from build123d import *

# Parameters (mm, degrees)
SKETCH2_W           = 50
SKETCH2_H           = 50
BOSS_EXTRUDE1_DEPTH = 50
CUT_EXTRUDE2_REACH  = 88.603
SKETCH5_R           = 2.1
CUT_EXTRUDE3_REACH  = 88.603
SKETCH6_R           = 15.5


with BuildPart() as part:
    # Sketch2 → Boss-Extrude1 (new body)
    with BuildSketch(Plane.XY):
        with Locations((25, 25)):
            Rectangle(SKETCH2_W, SKETCH2_H)
    extrude(amount=BOSS_EXTRUDE1_DEPTH)

    # Sketch5 → Cut-Extrude2 (cut, up to next)
    with BuildSketch(Plane(origin=(0, 50, 0), x_dir=(1, 0, 0), z_dir=(0, 1, 0)), mode=Mode.PRIVATE) as cut_extrude2_sk1:
        with Locations(Location((7.5, -7.5, 0), (0, 0, 270))):
            Circle(SKETCH5_R)
    cut_extrude2_tool1 = extrude(cut_extrude2_sk1.sketch, amount=-CUT_EXTRUDE2_REACH, mode=Mode.PRIVATE) & part.part
    # Sketch5 → Cut-Extrude2 (cut, up to next)
    with BuildSketch(Plane(origin=(0, 50, 0), x_dir=(1, 0, 0), z_dir=(0, 1, 0)), mode=Mode.PRIVATE) as cut_extrude2_sk2:
        with Locations(Location((42.5, -7.5, 0), (0, 0, 270))):
            Circle(SKETCH5_R)
    cut_extrude2_tool2 = extrude(cut_extrude2_sk2.sketch, amount=-CUT_EXTRUDE2_REACH, mode=Mode.PRIVATE) & part.part
    # Sketch5 → Cut-Extrude2 (cut, up to next)
    with BuildSketch(Plane(origin=(0, 50, 0), x_dir=(1, 0, 0), z_dir=(0, 1, 0)), mode=Mode.PRIVATE) as cut_extrude2_sk3:
        with Locations(Location((7.5, -42.5, 0), (0, 0, 270))):
            Circle(SKETCH5_R)
    cut_extrude2_tool3 = extrude(cut_extrude2_sk3.sketch, amount=-CUT_EXTRUDE2_REACH, mode=Mode.PRIVATE) & part.part
    # Sketch5 → Cut-Extrude2 (cut, up to next)
    with BuildSketch(Plane(origin=(0, 50, 0), x_dir=(1, 0, 0), z_dir=(0, 1, 0)), mode=Mode.PRIVATE) as cut_extrude2_sk4:
        with Locations(Location((42.5, -42.5, 0), (0, 0, 270))):
            Circle(SKETCH5_R)
    cut_extrude2_tool4 = extrude(cut_extrude2_sk4.sketch, amount=-CUT_EXTRUDE2_REACH, mode=Mode.PRIVATE) & part.part
    add(cut_extrude2_tool1.solids().sort_by_distance((7.5, 50, 7.5))[0], mode=Mode.SUBTRACT)
    add(cut_extrude2_tool2.solids().sort_by_distance((42.5, 50, 7.5))[0], mode=Mode.SUBTRACT)
    add(cut_extrude2_tool3.solids().sort_by_distance((7.5, 50, 42.5))[0], mode=Mode.SUBTRACT)
    add(cut_extrude2_tool4.solids().sort_by_distance((42.5, 50, 42.5))[0], mode=Mode.SUBTRACT)

    # Sketch6 → Cut-Extrude3 (cut, up to next)
    with BuildSketch(Plane(origin=(0, 50, 0), x_dir=(-1, 0, 0), z_dir=(0, 1, 0)), mode=Mode.PRIVATE) as cut_extrude3_sk1:
        with Locations(Location((-25, 25, 0), (0, 0, 90))):
            Circle(SKETCH6_R)
    cut_extrude3_tool1 = extrude(cut_extrude3_sk1.sketch, amount=-CUT_EXTRUDE3_REACH, mode=Mode.PRIVATE) & part.part
    add(cut_extrude3_tool1.solids().sort_by_distance((25, 50, 25))[0], mode=Mode.SUBTRACT)


solid = part.part
Input: part model. Units: mm. Frame: model coordinates. Give positions to 0.01 mm unless a question says otherwise; leave off trailing zeros. Write each loop counter-clockwise with the first axis right and the second up, starting at its lowest first coordinate (ties: lowest second). Pieces come first, ordered by that corner, then holes. Notation, with made-up numbers: M 15,2 L 37,2 A23 cw 37,10 Z; hole C 40,69 d3. An arc over 180 degrees is marked long. Use one line per item in the form item = value.
1. First-contact query: P1, Ø4, axis at x = 7.5, z = 7.5, coming from the +Y side. Flat tip, straight axial feed; report the tip coordinate or a pass-through.
Outcome:
P1 = through
2. Ray query, L1, parallel to X at y = 23, z = 7.5; L2, parallel to Z at x = 9, y = 48; L3, parallel to X at y = 31, z = 42. Return the intervals inside material, ascending.
Outcome:
L1 = 0 to 5.4, 9.6 to 40.4, 44.6 to 50
L2 = 0 to 6.03, 8.97 to 41.03, 43.97 to 50
L3 = 0 to 5.46, 9.54 to 40.46, 44.54 to 50
3. Cut plane C-C on x = 25. Return loops of the section in (y, z), and give its area (3 significant figures).
Outcome:
outline = M 0,0 L 50,0 L 50,9.5 L 0,9.5 Z; M 0,40.5 L 50,40.5 L 50,50 L 0,50 Z
area = 950 mm²
4. Cut plane A-A on z = 42.5. Return loops of the section in (x, y), and give its area (3 significant figures).
Outcome:
outline = M 0,0 L 5.4,0 L 5.4,50 L 0,50 Z; M 9.6,0 L 40.4,0 L 40.4,50 L 9.6,50 Z; M 44.6,0 L 50,0 L 50,50 L 44.6,50 Z
area = 2,080 mm²
5. Cut plane B-B on x = 7.5. Return loops of the section in (y, z), and give its area (3 significant figures).
Outcome:
outline = M 0,0 L 50,0 L 50,5.4 L 0,5.4 Z; M 0,9.6 L 50,9.6 L 50,40.4 L 0,40.4 Z; M 0,44.6 L 50,44.6 L 50,50 L 0,50 Z
area = 2,080 mm²
6. Mould query, pull axis Z, two halves, no side actions, for faces 1 (the face through (25, 25, 50)), 2 (the face through (50, 25, 25)), 3 (the face through (9.582, 25.35, 42.227)). Classes: released by +Z, released by -Z, zero draft, split by the parting line, or undercut.
Outcome:
face_1 = released by +Z
face_2 = zero draft
face_3 = undercut
7. Cut plane D-D on z = 25. Return loops of the section in (x, y).
Outcome:
outline = M 0,0 L 9.5,0 L 9.5,50 L 0,50 Z; M 40.5,0 L 50,0 L 50,50 L 40.5,50 Z
